from build123d import *

# Parameters (mm, degrees)
SKETCH1_R           = 5.9944
BOSS_EXTRUDE1_DEPTH = 2.54
SKETCH1_5_W         = 2.54
SKETCH1_5_H         = 101.6
REVOLVE3_ANGLE      = 10


with BuildPart() as part:
    # Sketch1 → Boss-Extrude1 (new body)
    with BuildSketch(Plane.XY):
        with BuildLine():
            Line((-48.26, 0), (-48.26, -101.6))
            add(Edge.make_bspline(
                [(-48.26, -101.6), (-44.589659251, -138.15139004), (-31.409290844, -178.560823803), (0, -200.66)],
                knots=[0, 0, 0, 0, 1, 1, 1, 1], degree=3))
            add(Edge.make_bspline(
                [(48.26, -101.6), (44.589659251, -138.15139004), (31.409290844, -178.560823803), (0, -200.66)],
                knots=[0, 0, 0, 0, 1, 1, 1, 1], degree=3))
            Line((48.26, -101.6), (48.26, 0))
            add(Edge.make_bspline(
                [(48.26, 0), (44.589659251, 36.55139004), (31.409290844, 76.960823803), (0, 99.06)],
                knots=[0, 0, 0, 0, 1, 1, 1, 1], degree=3))
            add(Edge.make_bspline(
                [(-48.26, 0), (-44.589659251, 36.55139004), (-31.409290844, 76.960823803), (0, 99.06)],
                knots=[0, 0, 0, 0, 1, 1, 1, 1], degree=3))
        make_face()
        with Locations((-30.48, -50.8)):
            Circle(SKETCH1_R, mode=Mode.SUBTRACT)
    extrude(amount=BOSS_EXTRUDE1_DEPTH)

    # Sketch1<5> → Revolve3 (revolve)
    with BuildSketch(Plane.XY):
        with Locations((46.99, -50.8)):
            Rectangle(SKETCH1_5_W, SKETCH1_5_H)
    revolve(axis=Axis((0, 0, 0), (0, -1, 0)), revolution_arc=REVOLVE3_ANGLE)


solid = part.part
The model under review builds one solid part; all positions refer to its coordinate system, in mm. Round coordinates to 2 decimals unless told otherwise and drop trailing zeros. Write each loop counter-clockwise with the first axis right and the second up, starting at its lowest first coordinate (ties: lowest second). Pieces come first, ordered by that corner, then holes. Notation, with made-up numbers: M 34,43.25 L 39,43.25 A24 cw 39,75.25 Z; hole C -23.5,35 d9. An arc over 180 degrees is marked long. Use a Markdown table: item, result. Add a question column.
Q1. We need section A-A, the plane y = -50.8. State the section outline as (x, z) points.
Q2. The part is to be moulded in two halves that separate along X. For faces 1 (the face through (45.422, -50.089, 5.211)), 2 (the face through (48, -50, 5)), 3 (the face through (-36.47, -50.54, 1.25)), say which applies: pulls with the +X half, pulls with the -X half, needs draft (parallel to the pull), parting line crosses it, or undercut.
Q3. To check wall thickness, follow line 1 (Z direction, x = -0.5, y = -186); line 2 (Y direction, x = -30.48, z = 0.9); line 3 (X direction, y = -67.5, z = 6.75). State the ranges of each line that lie inside material, in increasing order.
Q4. Insertion check: pin 1 (5 mm diameter, centred on x = 35.5, y = -83.5, fed in from +Z); pin 2 (3 mm diameter, centred on y = -75, z = 4.5, fed in from +X); pin 3 (2.5 mm diameter, centred on x = 46, z = 4.5, fed in from -Y). Each pin has a flat end and moves straight along its axis. Give the tip position at first contact, or say it passes through.
Q5. We need section C-C, the plane z = 6.5. State the section outline as (x, y) points.
Q6. We need section B-B, the plane y = -89. State the section outline as (x, z) points, plus the area to 3 significant figures.
Findings below:
| question | item | result |
|---|---|---|
| 1 | outline | M -48.26,0 L -36.47,0 L -36.47,2.54 L -48.26,2.54 Z; M -24.49,0 L 48.26,0 L 48.26,2.54 L 48.19,2.54 A48.26 ccw 47.53,8.38 L 45.03,7.94 A45.72 cw 45.65,2.54 L -24.49,2.54 Z |
| 2 | face 1 | pulls with the -X half |
| 2 | face 2 | pulls with the +X half |
| 2 | face 3 | undercut |
| 3 | line 1 | z = 0 to 2.54 |
| 3 | line 2 | y = -164.95 to -56.79, -44.81 to 63.35 |
| 3 | line 3 | x = 45.22 to 47.79 |
| 4 | pin 1 | stops at z = 2.54 |
| 4 | pin 2 | stops at x = 48.17 |
| 4 | pin 3 | stops at y = -101.6 |
| 5 | outline | M 45.26,-101.6 L 47.82,-101.6 L 47.82,0 L 45.26,0 Z |
| 6 | outline | M -48.26,0 L 48.26,0 L 48.26,2.54 L 48.19,2.54 A48.26 ccw 47.53,8.38 L 45.03,7.94 A45.72 cw 45.65,2.54 L -48.26,2.54 Z |
| 6 | area | 260 mm² |
